Input: part model. Units: mm. Frame: model coordinates. Give positions to 0.01 mm unless a question says otherwise; leave off trailing zeros. Loops run counter-clockwise (first coordinate to the right, second up) from the corner with the lowest first, then second, coordinate; pieces in that order, holes last.
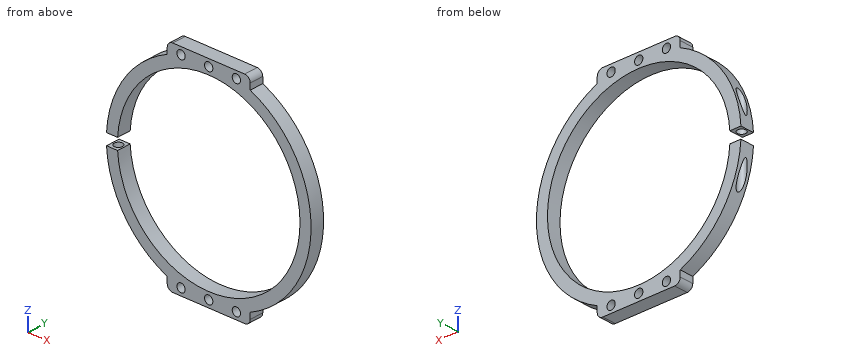
from build123d import *

# Parameters (mm, degrees)
CROQUIS1_R                 = 1.5
SALIENTE_EXTRUIR1_DEPTH    = 5
REDONDEO1_R                = 2
CORTAR_EXTRUIR1_DEPTH      = 20
CORTAR_EXTRUIR1_DEPTH_BACK = 15
CROQUIS3_R                 = 1.5


with BuildPart() as part:
    # Croquis1 → Saliente-Extruir1 (new body)
    with BuildSketch(Plane(origin=(0, 0, 0), x_dir=(1, 0, 0), z_dir=(0, 1, 0))):
        with BuildLine():
            Line((-32.939338184, -2), (-36.945906404, -2))
            ThreePointArc((-36.945906404, -2), (-30.459337304, -21.005446223), (-15, -33.823069051))
            Line((-15, -33.823069051), (-15, -38))
            Line((-15, -38), (15, -38))
            Line((15, -38), (15, -33.823069051))
            ThreePointArc((15, -33.823069051), (37, 0), (15, 33.823069051))
            Line((15, 33.823069051), (15, 38))
            Line((15, 38), (-15, 38))
            Line((-15, 38), (-15, 33.823069051))
            ThreePointArc((-15, 33.823069051), (-30.459337304, 21.005446223), (-36.945906404, 2))
            Line((-36.945906404, 2), (-32.939338184, 2))
            ThreePointArc((-32.939338184, 2), (33, 0), (-32.939338184, -2))
        make_face()
        with Locations(Location((0, -35.5, 0), (0, 0, 270))):
            Circle(CROQUIS1_R, mode=Mode.SUBTRACT)
        with Locations(Location((10, -35.5, 0), (0, 0, 270))):
            Circle(CROQUIS1_R, mode=Mode.SUBTRACT)
        with Locations(Location((-10, -35.5, 0), (0, 0, 270))):
            Circle(CROQUIS1_R, mode=Mode.SUBTRACT)
        with Locations(Location((10, 35.5, 0), (0, 0, 270))):
            Circle(CROQUIS1_R, mode=Mode.SUBTRACT)
        with Locations(Location((0, 35.5, 0), (0, 0, 270))):
            Circle(CROQUIS1_R, mode=Mode.SUBTRACT)
        with Locations(Location((-10, 35.5, 0), (0, 0, 270))):
            Circle(CROQUIS1_R, mode=Mode.SUBTRACT)
    extrude(amount=SALIENTE_EXTRUIR1_DEPTH)

    # Redondeo1
    redondeo1_edges = [part.edges().sort_by_distance(p)[0] for p in [
        (15, 2.5, 38),
        (-15, 2.5, 38),
        (-15, 2.5, -38),
        (15, 2.5, -38),
    ]]
    fillet(redondeo1_edges, radius=REDONDEO1_R)

    # Croquis3 → Cortar-Extruir1 (cut, two sides: drawn at the far end of the back side and taken through both)
    with BuildSketch(Plane(origin=(0, 0, 2), x_dir=(-1, 0, 0), z_dir=(0, 0, -1)).offset(-CORTAR_EXTRUIR1_DEPTH_BACK)):
        with Locations(Location((34.942622294, 2.5, 0), (0, 0, 180))):
            Circle(CROQUIS3_R)
    extrude(amount=CORTAR_EXTRUIR1_DEPTH + CORTAR_EXTRUIR1_DEPTH_BACK, mode=Mode.SUBTRACT)


solid = part.part
(1) Cut plane A-A (x = 0). Return the cut outline in (y, z), and give its area (3 significant figures).
Values follow:
outline: (0, -38) - (5, -38) - (5, -37) - (0, -37) - close; (0, -34) - (5, -34) - (5, -33) - (0, -33) - close; (0, 33) - (5, 33) - (5, 34) - (0, 34) - close; (0, 37) - (5, 37) - (5, 38) - (0, 38) - close
area: 20.0 mm2
(2) Cut plane B-B (z = -4). Return the cut outline in (x, y).
Values follow:
outline: (-36.78, 0) - (-32.76, 0) - (-32.76, 5) - (-36.78, 5) - close; (32.76, 0) - (36.78, 0) - (36.78, 5) - (32.76, 5) - close; hole circle Ø3 at (-34.94, 2.5)
(3) Ray query, probe 1 along X at (y, z) = (1.1, 35.5); probe 2 along Z at (x, y) = (-11, 0.95); probe 3 along X at (y, z) = (4.35, 11.5). Return the intervals inside material, ascending.
Values follow:
probe 1: x = -15 to -11.5, -8.5 to -1.5, 1.5 to 8.5, 11.5 to 15
probe 2: z = -38 to -36.62, -34.38 to -31.11, 31.11 to 34.38, 36.62 to 38
probe 3: x = -35.17 to -30.93, 30.93 to 35.17
(4) Pin query (flat end, axial travel): pin 1 Ø1.2 at (x, y) = (-34, 1.5) entering from +Z; pin 2 Ø2 at (y, z) = (1.5, -21.5) entering from -X; pin 3 Ø1 at (y, z) = (1, -25.5) entering from +X. Return the tip coordinate at first contact, or that it passes through.
Values follow:
pin 1: stops at z = 15.92
pin 2: stops at x = -30.8
pin 3: stops at x = 27.28
(5) Cut plane C-C (z = 23.5). Return the cut outline in (x, y), and give its area (3 significant figures).
Values follow:
outline: (-28.58, 0) - (-23.17, 0) - (-23.17, 5) - (-28.58, 5) - close; (23.17, 0) - (28.58, 0) - (28.58, 5) - (23.17, 5) - close
area: 54.1 mm2
(6) Cut plane D-D (x = -18.5). Return the cut outline in (y, z).
Values follow:
outline: (0, -32.04) - (5, -32.04) - (5, -27.33) - (0, -27.33) - close; (0, 27.33) - (5, 27.33) - (5, 32.04) - (0, 32.04) - close
